```python
from build123d import *

# Parameters (mm, degrees)
SKETCH1_W           = 13.97
SKETCH1_H           = 20.1041
BOARD_OUTLINE_DEPTH = 0.9144
SKETCH2_R           = 0.0762
NPTH_DEPTH          = 1.9144
SKETCH3_R           = 0.405
SKETCH3_R_2         = 1.27
PTH_DEPTH           = 1.9144


with BuildPart() as part:
    # Sketch1 → Board_Outline (new body)
    with BuildSketch(Plane.XY):
        with Locations((6.985, 10.05205)):
            Rectangle(SKETCH1_W, SKETCH1_H)
    extrude(amount=BOARD_OUTLINE_DEPTH)

    # Sketch2 → NPTH (cut, through all)
    with BuildSketch(Plane.XY):
        with Locations((10.7696, 3.683)):
            Circle(SKETCH2_R)
        with Locations((12.954, 16.891)):
            Circle(SKETCH2_R)
        with Locations((1.0668, 17.653)):
            Circle(SKETCH2_R)
        with Locations((1.4478, 14.605)):
            Circle(SKETCH2_R)
        with Locations((1.397, 13.8176)):
            Circle(SKETCH2_R)
        with Locations((4.1148, 11.5316)):
            Circle(SKETCH2_R)
        with Locations((4.3942, 11.049)):
            Circle(SKETCH2_R)
        with Locations((4.5466, 10.5156)):
            Circle(SKETCH2_R)
        with Locations((4.699, 9.9822)):
            Circle(SKETCH2_R)
        with Locations((4.8514, 9.4488)):
            Circle(SKETCH2_R)
        with Locations((5.0292, 8.9408)):
            Circle(SKETCH2_R)
        with Locations((5.461, 11.2522)):
            Circle(SKETCH2_R)
        with Locations((5.6134, 10.7188)):
            Circle(SKETCH2_R)
        with Locations((5.7658, 10.1854)):
            Circle(SKETCH2_R)
        with Locations((5.9182, 9.652)):
            Circle(SKETCH2_R)
        with Locations((6.0706, 9.1186)):
            Circle(SKETCH2_R)
        with Locations((6.223, 8.5852)):
            Circle(SKETCH2_R)
        with Locations((6.3754, 8.0518)):
            Circle(SKETCH2_R)
        with Locations((6.6802, 7.5946)):
            Circle(SKETCH2_R)
        with Locations((12.5476, 14.605)):
            Circle(SKETCH2_R)
        with Locations((12.7, 13.5128)):
            Circle(SKETCH2_R)
        with Locations((9.8806, 11.557)):
            Circle(SKETCH2_R)
        with Locations((9.4996, 11.0998)):
            Circle(SKETCH2_R)
        with Locations((9.3472, 10.5664)):
            Circle(SKETCH2_R)
        with Locations((9.1948, 10.033)):
            Circle(SKETCH2_R)
        with Locations((9.0424, 9.4996)):
            Circle(SKETCH2_R)
        with Locations((8.89, 8.9662)):
            Circle(SKETCH2_R)
        with Locations((8.4328, 11.2522)):
            Circle(SKETCH2_R)
        with Locations((8.2804, 10.7188)):
            Circle(SKETCH2_R)
        with Locations((8.128, 10.1854)):
            Circle(SKETCH2_R)
        with Locations((7.9756, 9.652)):
            Circle(SKETCH2_R)
        with Locations((7.8232, 9.1186)):
            Circle(SKETCH2_R)
        with Locations((7.6708, 8.5852)):
            Circle(SKETCH2_R)
        with Locations((7.5184, 8.0518)):
            Circle(SKETCH2_R)
        with Locations((7.2136, 7.5946)):
            Circle(SKETCH2_R)
        with Locations((1.7018, 7.4676)):
            Circle(SKETCH2_R)
        with Locations((1.27, 7.7978)):
            Circle(SKETCH2_R)
        with Locations((0.8382, 7.4676)):
            Circle(SKETCH2_R)
        with Locations((12.954, 17.5514)):
            Circle(SKETCH2_R)
        with Locations((1.0668, 16.891)):
            Circle(SKETCH2_R)
        with Locations((9.652, 5.715)):
            Circle(SKETCH2_R)
        with Locations((3.8608, 5.715)):
            Circle(SKETCH2_R)
    extrude(amount=NPTH_DEPTH, mode=Mode.SUBTRACT)

    # Sketch3 → PTH (cut, through all)
    with BuildSketch(Plane.XY):
        with Locations((12.83, 11.68)):
            Circle(SKETCH3_R)
        with Locations((2.74, 2.87)):
            Circle(SKETCH3_R_2)
        with Locations((1.17, 11.68)):
            Circle(SKETCH3_R)
    extrude(amount=PTH_DEPTH, mode=Mode.SUBTRACT)


solid = part.part
```
Design review of the part built by this model. Coordinates are the model's own, in mm. Coordinates: 2 decimals unless noted, no trailing zeros. Order: outer loops, then holes, each group sorted by start corner. A loop starts at its lowest first (then second) coordinate and runs counter-clockwise, first axis right, second up. Notation, with made-up numbers: (72, 78.5) - (87, 78.5) arc R17 ccw to (87, 94.5) - close; hole circle Ø6 at (-11.75, 76). An arc over 180 degrees is marked (long way). Answer in a Markdown table with one row per item.
(1) Wall thickness on line 1 along Y through (x, z) = (12.83, 0.5) (3 decimals); line 2 along Y through (x, z) = (2.75, 0.2); line 3 along X through (y, z) = (2.87, 0.25): over which ranges is each line inside the solid? List them lowest first. Write a range as from..to.
Checked values:
| item | result |
|---|---|
| line 1 | 0..11.275, 12.085..20.104 |
| line 2 | 0..1.6, 4.14..20.1 |
| line 3 | 0..1.47, 4.01..13.97 |
(2) Consider section A-A on y = 2.87. State the section outline as (x, z) points.
Checked values:
| item | result |
|---|---|
| outline | (0, 0) - (1.47, 0) - (1.47, 0.91) - (0, 0.91) - close; (4.01, 0) - (13.97, 0) - (13.97, 0.91) - (4.01, 0.91) - close |
(3) Consider section B-B on x = 2.74. State the section outline as (y, z) points, plus the area to 3 significant figures.
Checked values:
| item | result |
|---|---|
| outline | (0, 0) - (1.6, 0) - (1.6, 0.91) - (0, 0.91) - close; (4.14, 0) - (20.1, 0) - (20.1, 0.91) - (4.14, 0.91) - close |
| area | 16.1 mm^2 |
(4) Consider section C-C on z = 0.65. Give the number of separate pieces and of enclosed holes in the cut face, plus the area to 3 significant figures.
Checked values:
| item | result |
|---|---|
| separate pieces | 1 |
| enclosed holes | 45 |
| area | 274 mm^2 |
(5) The part is to be moulded in two halves that separate along Y. For faces 1 (the flat face through (13.97, 9.9, 0.5)), 2 (the flat face through (6.9, 20.104, 0.5)), 3 (the cylindrical face through (2.57, 4.13, 0.45)), say which applies: released by +Y, released by -Y, zero draft, split by the parting line, or undercut.
Checked values:
| item | result |
|---|---|
| face 1 | zero draft |
| face 2 | released by +Y |
| face 3 | undercut |
